Check sheet for the modelled part. Datum: model origin and axes. Units: mm. Give positions to 0.01 mm unless a question says otherwise; leave off trailing zeros. Loops run counter-clockwise (first coordinate to the right, second up) from the corner with the lowest first, then second, coordinate; pieces in that order, holes last. Notation, with made-up numbers: M 40.5,27 L 48.5,27 A11 ccw 48.5,45 Z; hole C -22.5,49 d3. An arc over 180 degrees is marked long. Write each question's results on one line, items separated by ' | '. Start each with the question number.
1. Sectioned sample at D-D on y = -12. Record the cut outline in (x, z).
2. Sectioned sample at C-C on x = 12.5. Record the cut outline in (y, z), and give its area (3 significant figures).
3. Draft check along X on faces 1 (the cylindrical face through (19.89, -9.06, 20.54)), 2 (the flat face through (0, -22, 41.656)), 3 (the flat face through (20.828, -17, 21)), 4 (the flat face through (-20.828, -17, 21)). Enter one of: pulls with the +X half, pulls with the -X half, needs draft (parallel to the pull), parting line crosses it, or undercut.
4. Go/stop test with a flat-tipped pin: pin 1 (3 mm diameter, centred on x = 12.5, y = -15, fed in from +Z). Record where the tip stops, or that it passes through.
5. Sectioned sample at B-B on z = 33.5. Record the cut outline in (x, y), and give its area (3 significant figures).
6. Sectioned sample at A-A on y = -19.25. Record the cut outline in (x, z).
7. Material ranges on line 1 along X through (y, z) = (-12, 5); line 2 along X through (y, z) = (-10.5, 38); line 3 along Y through (x, z) = (0.5, 33), recorded low to high.
```python
from build123d import *

# Parameters (mm, degrees)
BOSS_EXTRUDE1_DEPTH = 41.656


with BuildPart() as part:
    # Sketch1 → Boss-Extrude1 (new body)
    with BuildSketch(Plane.XY):
        with BuildLine():
            Line((-20.828, -10.28621602), (-20.828, -24.308623206))
            Line((-20.828, -24.308623206), (20.828, -24.308623206))
            Line((20.828, -24.308623206), (20.828, -10.28621602))
            ThreePointArc((20.828, -10.28621602), (19.862459196, -9.053250246), (18.433977011, -9.695054179))
            ThreePointArc((18.433977011, -9.695054179), (0, -20.828), (-18.433977011, -9.695054179))
            ThreePointArc((-18.433977011, -9.695054179), (-19.862459196, -9.053250246), (-20.828, -10.28621602))
        make_face()
    extrude(amount=BOSS_EXTRUDE1_DEPTH)


solid = part.part
```
Output values:
1) outline: M -20.83,0 L -17.02,0 L -17.02,41.66 L -20.83,41.66 Z; M 17.02,0 L 20.83,0 L 20.83,41.66 L 17.02,41.66 Z
2) outline: M -24.31,0 L -16.66,0 L -16.66,41.66 L -24.31,41.66 Z | area: 319 mm2
3) face 1: undercut | face 2: needs draft | face 3: pulls with the +X half | face 4: pulls with the -X half
4) pin 1: z = 41.66
5) outline: M -20.83,-24.31 L 20.83,-24.31 L 20.83,-10.29 A1.27 ccw 18.43,-9.7 A20.83 cw -18.43,-9.7 A1.27 ccw -20.83,-10.29 Z | area: 318 mm2
6) outline: M -20.83,0 L -7.95,0 L -7.95,41.66 L -20.83,41.66 Z; M 7.95,0 L 20.83,0 L 20.83,41.66 L 7.95,41.66 Z
7) line 1: -20.83 to -17.02, 17.02 to 20.83 | line 2: -20.83 to -17.99, 17.99 to 20.83 | line 3: -24.31 to -20.82
